```python
from build123d import *

# Parameters (mm, degrees)
SKETCH1_W           = 18.7
SKETCH1_H           = 3.2
BOSS_EXTRUDE1_DEPTH = 6.35
SKETCH2_R           = 1.35
CUT_EXTRUDE1_DEPTH  = 6.35


with BuildPart() as part:
    # Sketch1 → Boss-Extrude1 (new body)
    with BuildSketch(Plane(origin=(0, 0, 0), x_dir=(1, 0, 0), z_dir=(0, 1, 0))):
        Polygon((70, -86.602540378), (110, -17.320508076), (40, 103.923048454), (-40, 103.923048454), (-110, -17.320508076), (-70, -86.602540378), align=None)
        Polygon((-94.671350353, -8.470508076), (-85.321350353, -24.665183126), (-88.092631645, -26.265183126), (-97.442631645, -10.070508076), align=None, mode=Mode.SUBTRACT)
        Polygon((-57.442631645, -79.352540378), (-54.671350353, -77.752540378), (-64.021350353, -61.557865328), (-66.792631645, -63.157865328), align=None, mode=Mode.SUBTRACT)
        Polygon((54.671350353, -77.752540378), (64.021350353, -61.557865328), (66.792631645, -63.157865328), (57.442631645, -79.352540378), align=None, mode=Mode.SUBTRACT)
        Polygon((97.442631645, -10.070508076), (94.671350353, -8.470508076), (85.321350353, -24.665183126), (88.092631645, -26.265183126), align=None, mode=Mode.SUBTRACT)
        with Locations((30.65, 87.823048454)):
            Rectangle(SKETCH1_W, SKETCH1_H, mode=Mode.SUBTRACT)
        with Locations((-30.65, 87.823048454)):
            Rectangle(SKETCH1_W, SKETCH1_H, mode=Mode.SUBTRACT)
    extrude(amount=BOSS_EXTRUDE1_DEPTH)

    # Sketch2 → Cut-Extrude1 (cut)
    with BuildSketch(Plane(origin=(0, 6.35, 0), x_dir=(1, 0, 0), z_dir=(0, 1, 0))):
        with Locations(Location((-24.5, -60.102540378, 0), (0, 0, 270))):
            Circle(SKETCH2_R)
        with Locations(Location((24.5, -60.102540378, 0), (0, 0, 270))):
            Circle(SKETCH2_R)
        with Locations(Location((24.5, -2.102540378, 0), (0, 0, 270))):
            Circle(SKETCH2_R)
        with Locations(Location((-24.5, -2.102540378, 0), (0, 0, 270))):
            Circle(SKETCH2_R)
    extrude(amount=-CUT_EXTRUDE1_DEPTH, mode=Mode.SUBTRACT)


solid = part.part
```
The model under review builds one solid part; all positions refer to its coordinate system, in mm. A direction names the side the tool comes from. Round coordinates to 2 decimals unless told otherwise and drop trailing zeros. Write each loop counter-clockwise with the first axis right and the second up, starting at its lowest first coordinate (ties: lowest second). Pieces come first, ordered by that corner, then holes. Notation, with made-up numbers: (-2.75, -18.5) -> (52.25, -18.5) arc R16 cw to (52.25, -9.5) -> close; hole circle Ø3 at (74, 50). An arc over 180 degrees is marked (long way). Use CSV: the item, a comma, the result in double quotes.
Q1. Consider section A-A (x = 32.5). Give the boundary of the cut face in (y, z), then the cut area to 3 significant figures.
Checks:
outline,"(0, -103.92) -> (6.35, -103.92) -> (6.35, -89.42) -> (0, -89.42) -> close; (0, -86.22) -> (6.35, -86.22) -> (6.35, 86.6) -> (0, 86.6) -> close"
area,"1,190 mm²"
Q2. Consider section B-B (y = 2). State how many separate pieces and enclosed holes the cut face has, then the cut area to 3 significant figures.
Checks:
separate pieces,"1"
enclosed holes,"10"
area,"30,300 mm²"
Q3. To check wall thickness, follow probe 1 along Z at (x, y) = (-37.5, 5.25); probe 2 along X at (y, z) = (0.75, 2.5); probe 3 along X at (y, z) = (0.75, 65). State the ranges of each line that lie inside material, in increasing order. Write a range as [from, to].
Checks:
probe 1,"[-103.92, -89.42], [-86.22, 86.6]"
probe 2,"[-101.44, -25.79], [-23.21, 23.21], [25.79, 101.44]"
probe 3,"[-82.47, -65.73], [-62.03, 62.03], [65.73, 82.47]"
Q4. For pin 1 Ø1 at (y, z) = (1.5, -87.5) entering from -X; pin 2 Ø1.6 at (y, z) = (1.5, -87.5) entering from -X; pin 3 Ø1.5 at (y, z) = (1.5, 9) entering from +X, all flat-tipped, find the tip position at first contact; note any pin that passes through.
Checks:
pin 1,"x = -49.77"
pin 2,"x = -49.94"
pin 3,"x = 105.63"
Q5. Mouldability with a two-part tool opening along Z and no side actions: class faces 3 (the flat face through (-90.28, 3.13, 51.48)), 4 (the flat face through (-74.51, 3.13, -44.15)), 5 (the flat face through (31, 3, -86.223)) as released by +Z, released by -Z, zero draft, split by the parting line, or undercut.
Checks:
face 3,"released by +Z"
face 4,"released by -Z"
face 5,"undercut"
Q6. For faces 1 (the flat face through (31, 3, -89.423)), 2 (the flat face through (-1, 3, 86.603)), list the 3-axis set-ups (+Z, -Z, +X, -X, +Y, -Y) from which the entire face can be reached by the end or side of a thin tool; tool diameter is ignored.
Checks:
face 1,"+Y, -Y"
face 2,"+Z, +X, -X, +Y, -Y"
Q7. Consider section C-C (x = -61.5). Give the boundary of the cut face in (y, z), then the cut area to 3 significant figures.
Checks:
outline,"(0, -66.68) -> (6.35, -66.68) -> (6.35, 65.92) -> (0, 65.92) -> close; (0, 72.32) -> (6.35, 72.32) -> (6.35, 86.6) -> (0, 86.6) -> close"
area,"933 mm²"
